```python
from build123d import *

# Parameters (mm, degrees)
BASE_EXTRUSION_DEPTH    = 3
ESQUISSE2_R             = 2
ENL_V_MAT_EXTRU_1_DEPTH = 3
CHANFREIN1_SIZE         = 0.5


with BuildPart() as part:
    # Esquisse1 → Base-Extrusion (new body)
    with BuildSketch(Plane.XY):
        with BuildLine():
            Line((-10, 4), (10, 4))
            ThreePointArc((10, 4), (14, 0), (10, -4))
            Line((10, -4), (-10, -4))
            ThreePointArc((-10, -4), (-14, 0), (-10, 4))
        make_face()
    extrude(amount=BASE_EXTRUSION_DEPTH)

    # Esquisse2 → Enlèv. mat.-Extru.1 (cut)
    with BuildSketch(Plane.XY.offset(3)):
        with Locations(Location((0, 0, 0), (0, 0, 180))):
            Circle(ESQUISSE2_R)
    extrude(amount=-ENL_V_MAT_EXTRU_1_DEPTH, mode=Mode.SUBTRACT)

    # Chanfrein1
    chanfrein1_edges = [part.edges().sort_by_distance(p)[0] for p in [
        (0, -4, 0),
        (0, -4, 3),
        (14, 0, 0),
        (14, 0, 3),
        (-14, 0, 0),
        (-14, 0, 3),
        (0, 4, 0),
        (2, 0, 0),
        (0, 4, 3),
        (2, 0, 3),
    ]]
    chamfer(chanfrein1_edges, length=CHANFREIN1_SIZE)


solid = part.part
```
Could you check a few things on this model? Use its own coordinates, in mm. Round coordinates to 2 decimals unless told otherwise and drop trailing zeros. Loops run counter-clockwise (first coordinate to the right, second up) from the corner with the lowest first, then second, coordinate; pieces in that order, holes last.
Q1. I want a section at C-C (z = 2.25). Write out the boundary of the cut face in (x, y).
Q2. Please list where these lines run through material, in increasing order: L1, parallel to Y at x = 0, z = 1.45; L2, parallel to X at y = -1, z = 2.3; L3, parallel to X at y = 0.5, z = 0.95.
Q3. I want a section at D-D (x = -9.25). Write out the boundary of the cut face in (y, z), and give its area (3 significant figures).
Q4. I want a section at B-B (y = 0). Write out the boundary of the cut face in (x, z).
Q5. Thinking about a two-plate mould opening in X: for faces 1 (the flat face through (-3, 0, 0)), 2 (the cylindrical face through (0, 2, 2)), 3 (the conical face through (-13.64, -0.08, 0.14)), which applies, pulls with the +X half, pulls with the -X half, needs draft (parallel to the pull), parting line crosses it, or undercut?
Q6. I want a section at A-A (x = 0). Write out the boundary of the cut face in (y, z).
Answer below:
1. outline: (-10, -4) - (10, -4) arc R4 ccw to (10, 4) - (-10, 4) arc R4 ccw to start; hole circle Ø4 at (0, 0)
2. L1: y = -4 to -2, 2 to 4
2. L2: x = -13.87 to -1.73, 1.73 to 13.87
2. L3: x = -13.97 to -1.94, 1.94 to 13.97
3. outline: (-4, 0.5) - (-3.5, 0) - (3.5, 0) - (4, 0.5) - (4, 2.5) - (3.5, 3) - (-3.5, 3) - (-4, 2.5) - close
3. area: 23.5 mm2
4. outline: (-14, 0.5) - (-13.5, 0) - (-2.5, 0) - (-2, 0.5) - (-2, 2.5) - (-2.5, 3) - (-13.5, 3) - (-14, 2.5) - close; (2, 0.5) - (2.5, 0) - (13.5, 0) - (14, 0.5) - (14, 2.5) - (13.5, 3) - (2.5, 3) - (2, 2.5) - close
5. face 1: needs draft
5. face 2: undercut
5. face 3: pulls with the -X half
6. outline: (-4, 0.5) - (-3.5, 0) - (-2.5, 0) - (-2, 0.5) - (-2, 2.5) - (-2.5, 3) - (-3.5, 3) - (-4, 2.5) - close; (2, 0.5) - (2.5, 0) - (3.5, 0) - (4, 0.5) - (4, 2.5) - (3.5, 3) - (2.5, 3) - (2, 2.5) - close
